Geometry check sheet. Reference: the model listing, model coordinates, mm. A direction names the side the tool comes from. Coordinates: 2 decimals unless noted, no trailing zeros. Write each loop counter-clockwise with the first axis right and the second up, starting at its lowest first coordinate (ties: lowest second). Pieces come first, ordered by that corner, then holes. Notation, with made-up numbers: (-37.5, -40) -> (-24.5, -40) arc R14 ccw to (-24.5, -24) -> close; hole circle Ø4 at (79, 45.25). An arc over 180 degrees is marked (long way). Answer in a Markdown table with one row per item. Add a question column.
Q1. Section check D-D, the plane z = 33. Record the boundary of the cut face in (x, y), and give its area (3 significant figures).
Q2. Gauge pin test, flat ends, axial feed: P1, Ø4, axis at x = 318.5, y = -7, coming from the -Z side; P2, Ø6, axis at x = -168, z = -287, coming from the +Y side; P3, Ø6, axis at x = 2.5, y = -28.5, coming from the -Z side. Record the tip position at first contact, or that the pin passes through.
Q3. Section check B-B, the plane x = 0. Record the boundary of the cut face in (y, z), and give its area (4 significant figures).
Q4. Thickness scan on line 1 (Y direction, x = 0, z = -160.5); line 2 (X direction, y = 100, z = -31.5); line 3 (Y direction, x = -60, z = -289.5). Record the ranges inside material, lowest first.
Q5. Section check A-A, the plane z = -166. Record the boundary of the cut face in (x, y).
Q6. Section check C-C, the plane y = 100.5. Record the boundary of the cut face in (x, z), and give its area (3 significant figures).
Q7. Tool access check on faces 1 (the face through (13, 202, 0)), 2 (the face through (-259.808, 6, 39)). Record the directions out of +Z, -Z, +X, -X, +Y, -Y that give a thin tool (end or side, any length) a straight path to the whole face; none if there is none.
Autodesk Fusion 360 part; units mm, degrees
sketch "Sketch2" plane through (0, 0, 0) normal (0, 0, 1) x (1, 0, 0)
  line L0 (519.6152, 0) -> (-259.8076, 450)
  line L1 (-259.8076, 450) -> (-259.8076, -450)
  line L2 (-259.8076, -450) -> (519.6152, 0)
  dimension "d4" = 900
extrude "Extrude2" add sketch "Sketch2" along normal blind 80
sketch "Sketch3" plane through (0, 0, 0) normal (0, 0, 1) x (1, 0, 0)
  circle A0 centre (0, 0) radius 125
  circle A1 centre (0, 0) radius 200
  circle A2 centre (0, 0) radius 175
  dimension "d7" = 250
  dimension "d8" = 400
  dimension "d9" = 350
extrude "Extrude3" add sketch "Sketch3" against normal blind 200 contours A0
extrude "Extrude4" add sketch "Sketch3" against normal blind 500 contours A1
extrude "Extrude5" cut 1 faces at (62.6805, -21.2553, -200) along direction (0, 0, 1) blind 200
extrude "Extrude6" add sketch "Sketch3" against normal blind 400 contours A0
extrude "Extrude7" cut 1 faces at (190.2705, -18.6303, -500) along direction (0, 0, 1) blind 100
extrude "Extrude8" add 1 faces at (190.2705, -18.6303, -400) along direction (0, 0, -1) blind 50
Calculated:
| question | item | result |
|---|---|---|
| 1 | outline | (-259.81, -450) -> (519.62, 0) -> (-259.81, 450) -> close |
| 1 | area | 351,000 mm² |
| 2 | P1 | stops at z = 0 |
| 2 | P2 | stops at y = 113.03 |
| 2 | P3 | stops at z = -400 |
| 3 | outline | (-300, 0) -> (-200, 0) -> (-200, -450) -> (-175, -450) -> (-175, 0) -> (-125, 0) -> (-125, -400) -> (125, -400) -> (125, 0) -> (175, 0) -> (175, -450) -> (200, -450) -> (200, 0) -> (300, 0) -> (300, 80) -> (-300, 80) -> close |
| 3 | area | 170,500 mm² |
| 4 | line 1 | y = -200 to -175, -125 to 125, 175 to 200 |
| 4 | line 2 | x = -173.21 to -143.61, -75 to 75, 143.61 to 173.21 |
| 4 | line 3 | y = -190.79 to -164.39, -109.66 to 109.66, 164.39 to 190.79 |
| 5 | outline | circle Ø400 at (0, 0); circle Ø250 at (0, 0); hole circle Ø350 at (0, 0) |
| 6 | outline | (-259.81, 0) -> (-172.92, 0) -> (-172.92, -450) -> (-143.26, -450) -> (-143.26, 0) -> (-74.33, 0) -> (-74.33, -400) -> (74.33, -400) -> (74.33, 0) -> (143.26, 0) -> (143.26, -450) -> (172.92, -450) -> (172.92, 0) -> (345.54, 0) -> (345.54, 80) -> (-259.81, 80) -> close |
| 6 | area | 135,000 mm² |
| 7 | face 1 | -Z |
| 7 | face 2 | +Z, -Z, -X, +Y, -Y |
